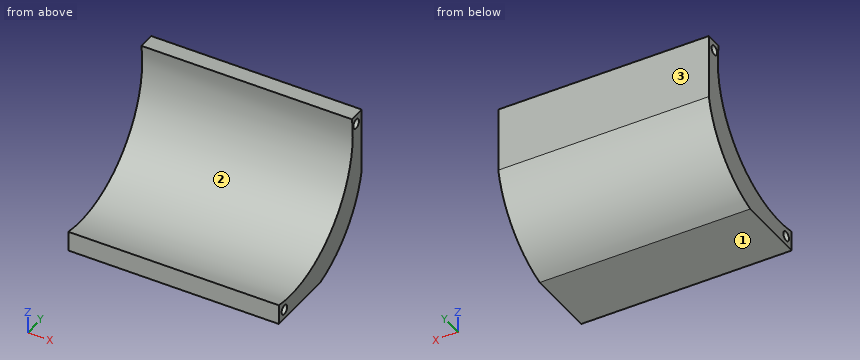
from build123d import *

# Parameters (mm, degrees)
F0_W     = 114.3
F0_H     = 76.2
F1_DEPTH = 76.2
F2_R     = 2.5527
F3_DEPTH = 114.3


# Not quite as in the source:
# - a feature names something its author has since deleted; it is built from what else it names


with BuildPart() as f1:
    # F0 (on Front) → F1 (new body)
    with BuildSketch(Plane.XZ):
        with Locations((0.8173113427, -2.9648756608)):
            Rectangle(F0_W, F0_H)
    extrude(amount=F1_DEPTH)

    # F2 (on face) → F3 (cut)
    with BuildSketch(Plane.YZ.offset(57.9673113427)):
        with Locations((-71.0946, -35.9848756608)):
            Circle(F2_R)
        with Locations((-5.08, 30.0551243392)):
            Circle(F2_R)
        with BuildLine():
            ThreePointArc((0, 0), (-13.3911011826, -25.7827653055), (-38.1, -41.0648756608))
            Line((-38.1, -41.0648756608), (0, -41.0648756608))
            Line((0, -41.0648756608), (0, 0))
        make_face()
        with BuildLine():
            Line((-76.2, 35.1351243392), (-76.2, -30.2226077765))
            ThreePointArc((-76.2, -30.2226077765), (-25.506077145, -15.1181602946), (-8.9947013184, 35.1351243392))
            Line((-8.9947013184, 35.1351243392), (-76.2, 35.1351243392))
        make_face()
    extrude(amount=-F3_DEPTH, mode=Mode.SUBTRACT)


solid = f1.part
Source: CAD feature listing. Evaluate the final solid. Frame: model axes, mm. Face numbers are marked on the shaded views. Give positions to 0.01 mm unless a question says otherwise; leave off trailing zeros. Write each loop counter-clockwise with the first axis right and the second up, starting at its lowest first coordinate (ties: lowest second). Pieces come first, ordered by that corner, then holes. Notation, with made-up numbers: M 76.5,88 L 88.5,88 A25 ccw 88.5,110 Z; hole C 35.25,-24 d8. An arc over 180 degrees is marked long. Answer as a JSON object with one key per item and string values.
Q1. Cut plane D-D, the plane z = -26. Return the cut outline in (x, y), then the cut area to 3 significant figures.
Geometry check:
{"outline": "M -56.33,-41.33 L 57.97,-41.33 L 57.97,-13.59 L -56.33,-13.59 Z", "area": "3,170 mm^2"}
Q2. Cut plane C-C, the plane y = -5.08. Return the cut outline in (x, z).
Geometry check:
{"outline": "M -56.33,-14.04 L 57.97,-14.04 L 57.97,27.5 L -56.33,27.5 Z; M -56.33,32.61 L 57.97,32.61 L 57.97,35.14 L -56.33,35.14 Z"}
Q3. Contact query for flat-ended pins moving along their axis: P1, Ø2, axis at x = 1.5, y = -13.5, coming from the +Z side; P2, Ø6, axis at x = 26.5, z = -10, coming from the +Y side; P3, Ø5, axis at x = 7.5, y = -21, coming from the +Z side; P4, Ø6, axis at y = -71.09, z = -35.98, coming from the +X side. Output: stop coordinate, or through.
Geometry check:
{"P1": "stops at z = 4.12", "P2": "stops at y = -1.99", "P3": "stops at z = -6.87", "P4": "stops at x = 57.97"}
Q4. Cut plane A-A, the plane x = 50.5. Return the cut outline in (y, z).
Geometry check:
{"outline": "M -76.2,-41.06 L -38.1,-41.06 A54.67 ccw 0,0 L 0,35.14 L -8.99,35.14 A57.07 cw -76.2,-30.22 Z; hole C -71.09,-35.98 d5.11; hole C -5.08,30.06 d5.11"}
Q5. Ray query, line 1 along Z through (x, y) = (-14, -3); line 2 along Z through (x, y) = (-4, -5.08); line 3 along Y through (x, z) = (30, -36.5). Return the intervals inside material, ascending.
Geometry check:
{"line 1": "z = -9.62 to 28.58, 31.53 to 35.14", "line 2": "z = -14.04 to 27.5, 32.61 to 35.14", "line 3": "y = -76.2 to -73.59, -68.59 to -27.12"}
Q6. Cut plane B-B, the plane y = -71. Return the cut outline in (x, z).
Geometry check:
{"outline": "M -56.33,-41.06 L 57.97,-41.06 L 57.97,-38.54 L -56.33,-38.54 Z; M -56.33,-33.43 L 57.97,-33.43 L 57.97,-30.99 L -56.33,-30.99 Z"}
Q7. Mould query, pull axis Y, two halves, no side actions, for the marked faces 1, 2 and 3. Classes: +Y half, -Y half, draft (parallel to the pull), parting line (faces both ways), or undercut.
Geometry check:
{"face 1": "draft", "face 2": "undercut", "face 3": "+Y half"}
